Work out the finished part from the listing and answer in its coordinate system (mm). Give positions to 0.01 mm unless a question says otherwise; leave off trailing zeros. Loops run counter-clockwise (first coordinate to the right, second up) from the corner with the lowest first, then second, coordinate; pieces in that order, holes last.
```python
from build123d import *

# Parameters (mm, degrees)
BOX_W     = 20
BOX_H     = 20
BOX_DEPTH = 9


with BuildPart() as cube:
    # Box → Box (new body)
    with BuildSketch(Plane(origin=(-10, -10, 1), x_dir=(1, 0, 0), z_dir=(0, 0, 1))):
        with Locations((10, 10)):
            Rectangle(BOX_W, BOX_H)
    extrude(amount=BOX_DEPTH)


with BuildPart() as obj1:
    # Sphere → Sphere (revolve)
    with BuildSketch(Plane(origin=(0, 0, 15), x_dir=(1, 0, 0), z_dir=(0, -1, 0))):
        with BuildLine():
            ThreePointArc((0, -8.6), (8.6, 0), (0, 8.6))
            Line((0, 8.6), (0, -8.6))
        make_face()
    revolve(axis=Axis((0, 0, 15), (0, 0, 1)))


with BuildPart() as obj2:
    # Sphere001 → Sphere001 (revolve)
    with BuildSketch(Plane(origin=(0, 0, 15), x_dir=(1, 0, 0), z_dir=(0, -1, 0))):
        with BuildLine():
            ThreePointArc((0, -10.6), (10.6, 0), (0, 10.6))
            Line((0, 10.6), (0, -10.6))
        make_face()
    revolve(axis=Axis((0, 0, 15), (0, 0, 1)))

    # Cut: cut obj1
    add(obj1.part, mode=Mode.SUBTRACT)

    # Cut001: cut Cube
    add(cube.part, mode=Mode.SUBTRACT)


solid = obj2.part
```
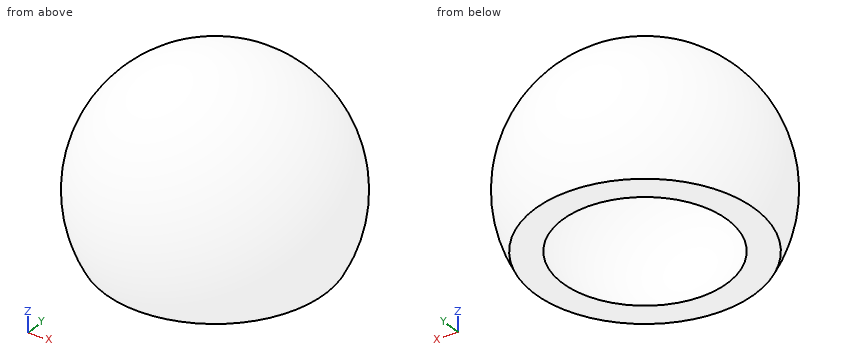
Q1. Section B-B on z = 16.5 is taken. Give the vertices of the cut face in (x, y), plus the area to 3 significant figures.
Q2. Section D-D on y = -2.5 is taken. Give the vertices of the cut face in (x, z), plus the area to 3 significant figures.
Q3. Section C-C on x = 3.5 is taken. Give the vertices of the cut face in (y, z), plus the area to 3 significant figures.
Q4. Section A-A on y = -8.25 is taken. Give the vertices of the cut face in (x, z).
Q5. Given pin 1 (4 mm diameter, centred on y = 1, z = 16.5, fed in from +X); pin 2 (1 mm diameter, centred on x = 5.5, y = 1.5, fed in from +Z); pin 3 (2 mm diameter, centred on y = -4.5, z = 17.5, fed in from +X); pin 4 (1 mm diameter, centred on x = 1, z = 19, fed in from -Y), each flat-ended and moving along its own axis, determine where each tip first touches the part or whether it passes through.
Q6. Consider line 1 along X through (y, z) = (5, 11.25); line 2 along X through (y, z) = (2.5, 16.5); line 3 along Y through (x, z) = (3.5, 11.75). Determine where each line is inside the solid, lowest interval first.
Check result:
1. outline: circle Ø20.99 at (0, 0); hole circle Ø16.94 at (0, 0)
1. area: 121 mm2
2. outline: (-9.01, 10) - (-6.54, 10) arc R8.23 cw (long way) to (6.54, 10) - (9.01, 10) arc R10.3 ccw (long way) to start
2. area: 82.2 mm2
3. outline: (-8.67, 10) - (-6.06, 10) arc R7.86 cw (long way) to (6.06, 10) - (8.67, 10) arc R10.01 ccw (long way) to start
3. area: 83.2 mm2
4. outline: (-4.39, 10) - (4.39, 10) arc R6.66 ccw (long way) to start; hole circle Ø4.86 at (0, 15)
5. pin 1: stops at x = 10.6
5. pin 2: stops at z = 24.24
5. pin 3: stops at x = 9.75
5. pin 4: stops at y = -9.96
6. line 1: x = -8.56 to -5.91, 5.91 to 8.56
6. line 2: x = -10.19 to -8.09, 8.09 to 10.19
6. line 3: y = -9.46 to -7.15, 7.15 to 9.46
